Model file for the job. Use its own axes, mm. A direction names the side the tool comes from. Give positions to 0.01 mm unless a question says otherwise; leave off trailing zeros. Loops run counter-clockwise (first coordinate to the right, second up) from the corner with the lowest first, then second, coordinate; pieces in that order, holes last. Notation, with made-up numbers: M 87.25,-21 L 93.25,-21 A17 cw 93.25,10 Z; hole C -11.5,52 d1. An arc over 180 degrees is marked long. Answer in a Markdown table with one row per item.
```python
from build123d import *

# Parameters (mm, degrees)
SKETCH_R     = 2.1082
SKETCH_W     = 90
SKETCH_H     = 90
PAD_DEPTH    = 8.89
SKETCH001_W  = 25.4
SKETCH001_H  = 25.4
SKETCH001_R  = 2.1463
PAD001_DEPTH = 8.89
PAD002_DEPTH = 8.89
PAD003_DEPTH = 0.889


with BuildPart() as part:
    # Sketch → Pad (new body)
    with BuildSketch(Plane.XY):
        Polygon((60, 60), (60, -60), (-60, -60), (-60, 60), (-60, 180), (60, 180), align=None)
        with Locations((-52.5, 52.5)):
            Circle(SKETCH_R, mode=Mode.SUBTRACT)
        with Locations((52.5, 52.5)):
            Circle(SKETCH_R, mode=Mode.SUBTRACT)
        with Locations((-52.5, -52.5)):
            Circle(SKETCH_R, mode=Mode.SUBTRACT)
        with Locations((52.5, -52.5)):
            Circle(SKETCH_R, mode=Mode.SUBTRACT)
        with Locations((-52.5, 172.5)):
            Circle(SKETCH_R, mode=Mode.SUBTRACT)
        with Locations((52.5, 172.5)):
            Circle(SKETCH_R, mode=Mode.SUBTRACT)
        with Locations((52.5, 67.5)):
            Circle(SKETCH_R, mode=Mode.SUBTRACT)
        with Locations((-52.5, 67.5)):
            Circle(SKETCH_R, mode=Mode.SUBTRACT)
        Rectangle(SKETCH_W, SKETCH_H, mode=Mode.SUBTRACT)
        with Locations((0, 120)):
            Rectangle(SKETCH_W, SKETCH_H, mode=Mode.SUBTRACT)
    extrude(amount=PAD_DEPTH)

    # Sketch001 (on Face24 of Pad) → Pad001 (join)
    with BuildSketch(Plane.XY.offset(8.89)):
        with Locations((-47.3, -72.7)):
            Rectangle(SKETCH001_W, SKETCH001_H)
        with Locations((-47.3, -72.7)):
            Circle(SKETCH001_R, mode=Mode.SUBTRACT)
        with Locations((47.3, -72.7)):
            Rectangle(SKETCH001_W, SKETCH001_H)
        with Locations((47.3, -72.7)):
            Circle(SKETCH001_R, mode=Mode.SUBTRACT)
    extrude(amount=-PAD001_DEPTH)

    # Sketch002 (on Face5 of Pad001) → Pad002 (join)
    with BuildSketch(Plane.XY.offset(8.89)):
        Polygon((-45, -40.7836), (-4.2164, 0), (-45, 40.7836), (-45, 45), (-40.7836, 45), (0, 4.2164), (40.7836, 45), (45, 45), (45, 40.7836), (4.2164, 0), (45, -40.7836), (45, -45), (40.7836, -45), (0, -4.2164), (-40.7836, -45), (-45, -45), align=None)
    extrude(amount=-PAD002_DEPTH)

    # Sketch003 (on Face5 of Pad001) → Pad003 (join)
    with BuildSketch(Plane.XY.offset(8.89)):
        Polygon((-45, 75), (-45, 79.2164), (-4.2164, 120), (-45, 160.7836), (-45, 165), (-40.7836, 165), (0, 124.2164), (40.7836, 165), (45, 165), (45, 160.7836), (4.2164, 120), (45, 79.2164), (45, 75), (40.7836, 75), (0, 115.7836), (-40.7836, 75), align=None)
    extrude(amount=-PAD003_DEPTH)


solid = part.part
```
(1) Flat gauge pin, fed straight in: P1, Ø3.5, axis at x = -52.5, y = -52.5, coming from the -Z side. Where does the tip first touch, or does it go through?
Established:
| item | result |
|---|---|
| P1 | passes through |
(2) Saw through at C-C, the plane x = 24. Give the cut face in (y, z), and give its area (3 significant figures).
Established:
| item | result |
|---|---|
| outline | M -60,0 L -45,0 L -45,8.89 L -60,8.89 Z; M -28.22,0 L -19.78,0 L -19.78,8.89 L -28.22,8.89 Z; M 19.78,0 L 28.22,0 L 28.22,8.89 L 19.78,8.89 Z; M 45,0 L 75,0 L 75,8.89 L 45,8.89 Z; M 91.78,8 L 100.22,8 L 100.22,8.89 L 91.78,8.89 Z; M 139.78,8 L 148.22,8 L 148.22,8.89 L 139.78,8.89 Z; M 165,0 L 180,0 L 180,8.89 L 165,8.89 Z |
| area | 698 mm2 |
(3) Mould opens along Y. For faces 1 (the flat face through (-34.6, -73, 5)), 2 (the flat face through (47, -85.4, 5)), 3 (the flat face through (45, 119, 4)) say: pulls with the +Y half, pulls with the -Y half, needs draft (parallel to the pull), parting line crosses it, or undercut.
Established:
| item | result |
|---|---|
| face 1 | needs draft |
| face 2 | pulls with the -Y half |
| face 3 | undercut |
(4) Which spindle directions (+Z, -Z, +X, -X, +Y, -Y) get a long thin tool onto all of the face, cutting with end or side? Do faces 4 (the flat face through (24.894, 20.677, 4.507)), 5 (the flat face through (34.6, -73, 5)), 6 (the flat face through (1, 49, 8.89)). Say none if no direction does.
Established:
| item | result |
|---|---|
| face 4 | +Z, -Z |
| face 5 | +Z, -Z, -Y |
| face 6 | +Z, +X, -X, +Y, -Y |
(5) Wall check: L1, parallel to Y at x = -52.5, z = 2; L2, parallel to Y at x = 47.3, z = 7.25; L3, parallel to Y at x = -6.5, z = 6.75. Give the ranges that are in metal, low to high.
Established:
| item | result |
|---|---|
| L1 | y = -85.4 to -54.61, -50.39 to 50.39, 54.61 to 65.39, 69.61 to 170.39, 174.61 to 180 |
| L2 | y = -85.4 to -74.85, -70.55 to 180 |
| L3 | y = -60 to -45, -10.72 to -2.28, 2.28 to 10.72, 45 to 75, 165 to 180 |
(6) Saw through at D-D, the plane y = 103. Give the cut face in (x, z), and give its area (3 significant figures).
Established:
| item | result |
|---|---|
| outline | M -60,0 L -45,0 L -45,8.89 L -60,8.89 Z; M -21.22,8 L -12.78,8 L -12.78,8.89 L -21.22,8.89 Z; M 12.78,8 L 21.22,8 L 21.22,8.89 L 12.78,8.89 Z; M 45,0 L 60,0 L 60,8.89 L 45,8.89 Z |
| area | 282 mm2 |
(7) Saw through at A-A, the plane z = 1.5. Count the separate pieces of the cut face and the enclosed holes in it, and give its area (3 significant figures).
Established:
| item | result |
|---|---|
| separate pieces | 1 |
| enclosed holes | 15 |
| area | 15,200 mm2 |
(8) Saw through at B-B, the plane y = -35. Give the cut face in (x, z).
Established:
| item | result |
|---|---|
| outline | M -60,0 L -45,0 L -45,8.89 L -60,8.89 Z; M -39.22,0 L -30.78,0 L -30.78,8.89 L -39.22,8.89 Z; M 30.78,0 L 39.22,0 L 39.22,8.89 L 30.78,8.89 Z; M 45,0 L 60,0 L 60,8.89 L 45,8.89 Z |
